```python
from build123d import *

# Parameters (mm, degrees)
SKETCH_1_R          = 1.9
EXTRUDE_1_DEPTH     = 2
SKETCH_2_R          = 1
EXTRUDE_2_DEPTH     = 8
CUT_EXTRUDE_1_DEPTH = 1


with BuildPart() as part:
    # 草图1 → 凸台-拉伸1 (new body)
    with BuildSketch(Plane.XY):
        Circle(SKETCH_1_R)
    extrude(amount=EXTRUDE_1_DEPTH)

    # 草图2 → 凸台-拉伸2 (add)
    with BuildSketch(Plane(origin=(0, 0, 0), x_dir=(-1, 0, 0), z_dir=(0, 0, -1))):
        Circle(SKETCH_2_R)
    extrude(amount=EXTRUDE_2_DEPTH)

    # 草图3 → 切除-拉伸1 (cut)
    with BuildSketch(Plane.XY.offset(2)):
        Polygon((-0.766222709, -0.403612141), (-0.033572987, -0.865374401), (0.732649722, -0.461762261), (0.766222709, 0.403612141), (0.033572987, 0.865374401), (-0.732649722, 0.461762261), align=None)
    extrude(amount=-CUT_EXTRUDE_1_DEPTH, mode=Mode.SUBTRACT)


solid = part.part
```
Verification items for the finished model (mm, model axes). A direction names the side the tool comes from. Round coordinates to 2 decimals unless told otherwise and drop trailing zeros. Order: outer loops, then holes, each group sorted by start corner. A loop starts at its lowest first (then second) coordinate and runs counter-clockwise, first axis right, second up.
1) Cross-section at B-B, the plane z = -5.5. Record the cut outline in (x, y).
Geometry says:
outline: circle Ø2 at (0, 0)
2) Draft check along X on faces 4 (the cylindrical face through (0, -1, -4)), 5 (the flat face through (-0.75, 0.04, 1.51)), 6 (the flat face through (0, 0, -8)), 7 (the flat face through (0.75, -0.04, 1.51)). Enter one of: +X half, -X half, draft (parallel to the pull), parting line (faces both ways), or undercut.
Geometry says:
face 4: parting line
face 5: undercut
face 6: draft
face 7: undercut
3) Material ranges on line 1 (Z direction, x = -0.3, y = -0.65); line 2 (Z direction, x = -1.1, y = 1.2); line 3 (Y direction, x = -0.05, z = -6.5), recorded low to high.
Geometry says:
line 1: z = -8 to 1
line 2: z = 0 to 2
line 3: y = -1 to 1
4) Cross-section at C-C, the plane x = -1.4. Record the cut outline in (y, z).
Geometry says:
outline: (-1.28, 0) - (1.28, 0) - (1.28, 2) - (-1.28, 2) - close
5) Cross-section at A-A, the plane y = 0.6. Record the cut outline in (x, z), plus the area to 3 significant figures.
Geometry says:
outline: (-1.8, 0) - (-0.8, 0) - (-0.8, -8) - (0.8, -8) - (0.8, 0) - (1.8, 0) - (1.8, 2) - (0.45, 2) - (0.45, 1) - (-0.47, 1) - (-0.47, 2) - (-1.8, 2) - close
area: 19.1 mm2
6) Tool access check on faces 1 (the flat face through (0, 0, 1)), 2 (the cylindrical face through (-1.9, 0.08, 0.99)), 3 (the flat face through (1, -1, 0)). Record the directions out of +Z, -Z, +X, -X, +Y, -Y that give a thin tool (end or side, any length) a straight path to the whole face; none if there is none.
Geometry says:
face 1: +Z
face 2: +Z, -Z
face 3: -Z
7) Cross-section at D-D, the plane y = 0. Record the cut outline in (x, z), plus the area to 3 significant figures.
Geometry says:
outline: (-1.9, 0) - (-1, 0) - (-1, -8) - (1, -8) - (1, 0) - (1.9, 0) - (1.9, 2) - (0.75, 2) - (0.75, 1) - (-0.75, 1) - (-0.75, 2) - (-1.9, 2) - close
area: 22.1 mm2
8) Depth check by flat-ended pin: pin 1 (1.5 mm diameter, centred on x = 1.5, z = -5.5, fed in from +Y). Enter the tip coordinate at first touch or a pass-through.
Geometry says:
pin 1: stops at y = 0.66
